Input: part model. Units: mm. Frame: model coordinates. Face numbers are marked on the shaded views. A direction names the side the tool comes from. Give positions to 0.01 mm unless a question says otherwise; leave off trailing zeros. Loops run counter-clockwise (first coordinate to the right, second up) from the corner with the lowest first, then second, coordinate; pieces in that order, holes last.
from build123d import *

# Parameters (mm, degrees)
BOSS_EXTRUDE1_DEPTH = 300
SKETCH3_R           = 25
CUT_EXTRUDE2_DEPTH  = 239
LPATTERN1_COUNT     = 2
LPATTERN1_PITCH     = 710
SKETCH4_R           = 112.5
SKETCH4_R_2         = 87.5
BOSS_EXTRUDE2_DEPTH = 170
SKETCH5_R           = 37.5
CUT_EXTRUDE3_DEPTH  = 170


with BuildPart() as part:
    # Sketch1 → Boss-Extrude1 (new body)
    with BuildSketch(Plane.XY):
        with BuildLine():
            Line((0, 0), (-167.5, 0))
            ThreePointArc((-167.5, 0), (-202.855339059, 14.644660941), (-217.5, 50))
            Line((-217.5, 50), (-217.5, 188))
            ThreePointArc((-217.5, 188), (-223.357864376, 202.142135624), (-237.5, 208))
            Line((-237.5, 208), (-475, 208))
            Line((-475, 208), (-475, 238))
            Line((-475, 238), (-237.5, 238))
            ThreePointArc((-237.5, 238), (-202.144660941, 223.355339059), (-187.5, 188))
            Line((-187.5, 188), (-187.5, 50))
            ThreePointArc((-187.5, 50), (-181.642135624, 35.857864376), (-167.5, 30))
            Line((-167.5, 30), (0, 30))
            Line((0, 30), (167.5, 30))
            ThreePointArc((167.5, 30), (181.642135624, 35.857864376), (187.5, 50))
            Line((187.5, 50), (187.5, 188))
            ThreePointArc((187.5, 188), (202.144660941, 223.355339059), (237.5, 238))
            Line((237.5, 238), (475, 238))
            Line((475, 238), (475, 208))
            Line((475, 208), (237.494317451, 208))
            ThreePointArc((237.494317451, 208), (223.35419134, 202.144144851), (217.494318258, 188.005683357))
            Line((217.494318258, 188.005683357), (217.455097442, 49.985791608))
            ThreePointArc((217.455097442, 49.985791608), (202.805414738, 14.639637872), (167.455099461, 0))
            Line((167.455099461, 0), (0, 0))
        make_face()
    extrude(amount=BOSS_EXTRUDE1_DEPTH)

    # Sketch3 → Cut-Extrude2 (cut, through all)
    with BuildSketch(Plane(origin=(0, 238, 0), x_dir=(1, 0, 0), z_dir=(0, 1, 0))):
        with Locations(Location((355, -150, 0), (0, 0, 180))):  # turned: the seam where the file's is
            Circle(SKETCH3_R)
    cut_extrude2 = extrude(amount=-CUT_EXTRUDE2_DEPTH, mode=Mode.SUBTRACT)

    # LPattern1: Cut-Extrude2 ×2
    with Locations(*[(-i * LPATTERN1_PITCH, 0, 0) for i in range(1, LPATTERN1_COUNT)]):
        add(cut_extrude2, mode=Mode.SUBTRACT)

    # Sketch4 → Boss-Extrude2 (add)
    with BuildSketch(Plane(origin=(0, 30, 0), x_dir=(1, 0, 0), z_dir=(0, 1, 0))):
        with Locations((0, -150)):
            Circle(SKETCH4_R)
        with Locations(Location((0, -150, 0), (0, 0, 180))):  # turned: the seam where the file's is
            Circle(SKETCH4_R_2, mode=Mode.SUBTRACT)
    extrude(amount=BOSS_EXTRUDE2_DEPTH)

    # Sketch5 → Cut-Extrude3 (cut)
    with BuildSketch(Plane(origin=(0, 30, 0), x_dir=(1, 0, 0), z_dir=(0, 1, 0))):
        with Locations(Location((0, -150, 0), (0, 0, 180))):  # turned: the seam where the file's is
            Circle(SKETCH5_R)
    extrude(amount=-CUT_EXTRUDE3_DEPTH, mode=Mode.SUBTRACT)


solid = part.part
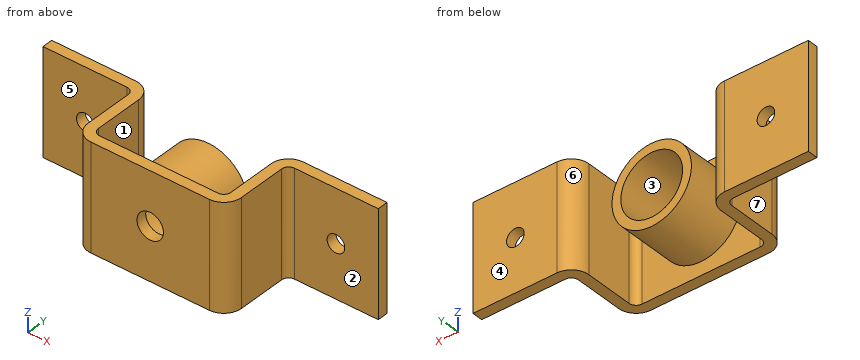
(1) Pin query (flat end, axial travel): pin 1 Ø2 at (x, y) = (50.5, 193) entering from +Z; pin 2 Ø2 at (x, z) = (208.5, 262) entering from -Y; pin 3 Ø4 at (y, z) = (69.5, 248) entering from +X. Return the tip coordinate at first contact, or that it passes through.
Values follow:
pin 1: stops at z = 251.02
pin 2: stops at y = 20.06
pin 3: stops at x = 217.46
(2) Cut plane B-B (y = 176.5). Return the cut outline in (x, z).
Values follow:
outline: (-217.5, 0) - (-187.5, 0) - (-187.5, 300) - (-217.5, 300) - close; circle Ø225 at (0, 150); (187.5, 0) - (217.49, 0) - (217.49, 300) - (187.5, 300) - close; hole circle Ø175 at (0, 150)
(3) Cut plane D-D (z = 150). Count the separate pieces of the cut face and the enclosed holes in it, and give its area (3 significant figures).
Values follow:
separate pieces: 4
enclosed holes: 0
area: 42,400 mm2
(4) Ray query, probe 1 along X at (y, z) = (152, 220); probe 2 along X at (y, z) = (39, 176) (3 decimals); probe 3 along Y at (x, z) = (-263.5, 252). Return the intervals inside material, ascending.
Values follow:
probe 1: x = -217.5 to -187.5, -88.07 to -52.5, 52.5 to 88.07, 187.5 to 217.48
probe 2: x = -216.275 to -184.203, -109.454 to -83.548, 83.548 to 109.454, 184.203 to 216.23
probe 3: y = 208 to 238
(5) Cut plane C-C (x = 0). Return the cut outline in (y, z).
Values follow:
outline: (0, 0) - (30, 0) - (30, 37.5) - (200, 37.5) - (200, 62.5) - (30, 62.5) - (30, 112.5) - (0, 112.5) - close; (0, 187.5) - (30, 187.5) - (30, 237.5) - (200, 237.5) - (200, 262.5) - (30, 262.5) - (30, 300) - (0, 300) - close
(6) Mould query, pull axis X, two halves, no side actions, for the marked faces 5, 6 and 7. Classes: +X half, -X half, draft (parallel to the pull), parting line (faces both ways), or undercut.
Values follow:
face 5: draft
face 6: undercut
face 7: -X half
(7) Reachability of the marked faces 1, 2, 3 and 4 from +Z, -Z, +X, -X, +Y, -Y: full face, straight path, thin tool, end or side. Return the list, or none.
Values follow:
face 1: +Z, -Z, +Y
face 2: +Z, -Z, +X, -Y
face 3: +Y
face 4: +Z, -Z, +X, -X, +Y
(8) Cut plane A-A (x = -355). Return the cut outline in (y, z).
Values follow:
outline: (208, 0) - (238, 0) - (238, 125) - (208, 125) - close; (208, 175) - (238, 175) - (238, 300) - (208, 300) - close
